Could you check a few things on this model? Use its own coordinates, in mm. Coordinates: 2 decimals unless noted, no trailing zeros. Write each loop counter-clockwise with the first axis right and the second up, starting at its lowest first coordinate (ties: lowest second). Pieces come first, ordered by that corner, then holes.
Item 1: If I drill on probe 1 along Z at (x, y) = (0, 1.4); probe 2 along Z at (x, y) = (1, 0.55); probe 3 along X at (y, z) = (0.25, -32.5), over which ranges is the centre line in solid material (lowest first)?
Item 2: Thinking about a two-plate mould opening in X: for faces 1 (the flat face through (-3.5, 1, -16)), 2 (the cylindrical face through (0.267, 0.986, -34.033)), 3 (the flat face through (0, 2, -16)), which applies, +X half, -X half, draft (parallel to the pull), parting line (faces both ways), or undercut?
Item 3: I want a section at B-B on y = 0.9. Please give me the cut outline in (x, z), then the cut area to 3 significant figures.
Item 4: I want a section at C-C on x = 1.5. Please give me the cut outline in (y, z).
Item 5: I want a section at A-A on x = 0. Please give me the cut outline in (y, z), then the cut area to 3 significant figures.
Autodesk Inventor part; units mm, degrees
ref_plane "YZ Plane" through (0, 0, 0) normal (1, 0, 0) x (0, 1, 0)
ref_plane "XZ Plane" through (0, 0, 0) normal (0, 1, 0) x (-1, 0, 0)
ref_plane "XY Plane" through (0, 0, 0) normal (0, 0, 1) x (1, 0, 0)
sketch "Sketch1" plane through (0, 0, 0) normal (0, 1, 0) x (-1, 0, 0)
  circle A0 centre (0, 0) radius 2.05
  circle A1 centre (0, -32) radius 2.05
  line L0 (0, 0) -> (0, -32) construction
  line L1 (-3.5, 0) -> (-3.5, -32)
  line L2 (3.5, -32) -> (3.5, 0)
  arc A2 (3.5, 0) -> (-3.5, 0) centre (0, 0) ccw
  arc A3 (-3.5, -32) -> (3.5, -32) centre (0, -32) ccw
  point P0 (0, -16)
  dimension "d1" = 4.1
  dimension "d2" = 4.1
  dimension "d3" = 7
extrude "Extrusion1" add sketch "Sketch1" along normal blind 2
properties part number "Micro_servo_frame_1"
Response values:
1. probe 1: z = -35.5 to -34.05, -29.95 to -2.05, 2.05 to 3.5
1. probe 2: z = -35.35 to -33.79, -30.21 to -1.79, 1.79 to 3.35
1. probe 3: x = -3.46 to -1.99, 1.99 to 3.46
2. face 1: -X half
2. face 2: undercut
2. face 3: draft
3. outline: (-3.5, -32) arc R3.5 ccw to (3.5, -32) - (3.5, 0) arc R3.5 ccw to (-3.5, 0) - close; hole circle Ø4.1 at (0, -32); hole circle Ø4.1 at (0, 0)
3. area: 236 mm2
4. outline: (0, -35.16) - (2, -35.16) - (2, -33.4) - (0, -33.4) - close; (0, -30.6) - (2, -30.6) - (2, -1.4) - (0, -1.4) - close; (0, 1.4) - (2, 1.4) - (2, 3.16) - (0, 3.16) - close
5. outline: (0, -35.5) - (2, -35.5) - (2, -34.05) - (0, -34.05) - close; (0, -29.95) - (2, -29.95) - (2, -2.05) - (0, -2.05) - close; (0, 2.05) - (2, 2.05) - (2, 3.5) - (0, 3.5) - close
5. area: 61.6 mm2
